The model under review builds one solid part; all positions refer to its coordinate system, in mm. A direction names the side the tool comes from. Give positions to 0.01 mm unless a question says otherwise; leave off trailing zeros. Loops run counter-clockwise (first coordinate to the right, second up) from the corner with the lowest first, then second, coordinate; pieces in that order, holes last. Notation, with made-up numbers: M 22.25,2.25 L 43.25,2.25 A10 ccw 43.25,20.25 Z; hole C 17.25,50.5 d2. An arc over 180 degrees is marked long. Write item = value, one per line. Start each with the question number.
1. For faces 5 (the face through (8.195, -7.969, -4.267)), 6 (the face through (8.85, 9.11, -4.27)), list the 3-axis set-ups (+Z, -Z, +X, -X, +Y, -Y) from which the entire face can be reached by the end or side of a thin tool; tool diameter is ignored.
2. We need section C-C on y = 10. Give the boundary of the cut face in (x, z), then the cut area to 3 significant figures.
3. We need section A-A on z = -69. Give the boundary of the cut face in (x, y), then the cut area to 3 significant figures.
4. Wall thickness on line 1 along X through (y, z) = (0, 137); line 2 along Y through (x, z) = (7, 35); line 3 along X through (y, z) = (-3, -20): over which ranges is each line inside the solid? List them lowest first. Write a range as from..to.
5. Draft analysis for pull direction Y (two halves, no side actions). For faces 1 (the face through (9.11, -8.85, -4.27)), 2 (the face through (-8.195, 7.969, -4.267)), 3 (the face through (-9.11, 8.85, -4.27)), 4 (the face through (-7.969, -8.195, -4.267)), state which applies: pulls with the +Y half, pulls with the -Y half, needs draft (parallel to the pull), parting line crosses it, or undercut.
6. We need section B-B on x = -5.5. Give the boundary of the cut face in (y, z).
7. For pin 1 (1 mm diameter, centred on y = 1.5, z = 204, fed in from -X); pin 2 (1.5 mm diameter, centred on x = -2, z = 186, fed in from -Y); pin 3 (12 mm diameter, centred on x = 6.5, z = -164.5, fed in from -Y), all flat-tipped, find the tip position at first contact; note any pin that passes through.
Autodesk Inventor part; units mm, degrees
ref_plane "YZ Plane" through (0, 0, 0) normal (1, 0, 0) x (0, 1, 0)
ref_plane "XZ Plane" through (0, 0, 0) normal (0, 1, 0) x (-1, 0, 0)
ref_plane "XY Plane" through (0, 0, 0) normal (0, 0, 1) x (1, 0, 0)
sketch "Sketch1" plane through (0, 0, 0) normal (0, 0, 1) x (1, 0, 0)
  line L0 (0, 17.9605) -> (17.9605, 0)
  line L1 (17.9605, 0) -> (0, -17.9605)
  line L2 (0, -17.9605) -> (-17.9605, 0)
  line L3 (-17.9605, 0) -> (0, 17.9605)
  line L4 (0, 17.9605) -> (0, -17.9605) construction
  line L5 (17.9605, 0) -> (-17.9605, 0) construction
  point P0 (0, 0)
  point P1 (0, 0)
  point P2 (0, 0)
  point P3 (0, 0)
  dimension "d2" = 25.4
  dimension "d3" = 25.4
extrude "Extrusion1" add sketch "Sketch1" along normal mid plane 609.6
shell "Shell1" thickness 1.27 removed faces 2 at (0, -5.9868, 304.8) at (0, -5.9868, -304.8)
properties part number "base_rail" material "Aluminum 6061"
Final values:
q1.face_5 = +Z, -Z
q1.face_6 = +Z, -Z, +X, +Y
q2.outline = M -7.96,-304.8 L -6.16,-304.8 L -6.16,304.8 L -7.96,304.8 Z; M 6.16,-304.8 L 7.96,-304.8 L 7.96,304.8 L 6.16,304.8 Z
q2.area = 2,190 mm²
q3.outline = M -17.96,0 L 0,-17.96 L 17.96,0 L 0,17.96 Z; hole M -16.16,0 L 0,-16.16 L 16.16,0 L 0,16.16 Z
q3.area = 123 mm²
q4.line_1 = -17.96..-16.16, 16.16..17.96
q4.line_2 = -10.96..-9.16, 9.16..10.96
q4.line_3 = -14.96..-13.16, 13.16..14.96
q5.face_1 = pulls with the -Y half
q5.face_2 = undercut
q5.face_3 = pulls with the +Y half
q5.face_4 = undercut
q6.outline = M -12.46,-304.8 L -10.66,-304.8 L -10.66,304.8 L -12.46,304.8 Z; M 10.66,-304.8 L 12.46,-304.8 L 12.46,304.8 L 10.66,304.8 Z
q7.pin_1 = -16.96
q7.pin_2 = -16.71
q7.pin_3 = -17.46
